Design review of the part built by this model. Coordinates are the model's own, in mm. A direction names the side the tool comes from. Coordinates: 2 decimals unless noted, no trailing zeros. Write each loop counter-clockwise with the first axis right and the second up, starting at its lowest first coordinate (ties: lowest second). Pieces come first, ordered by that corner, then holes. Notation, with made-up numbers: (-36, -20) - (-31, -20) arc R14 cw to (-31, -8) - close; hole circle Ø7 at (57.5, -1). An arc over 180 degrees is marked (long way). Use a Markdown table: item, result.
from build123d import *

# Parameters (mm, degrees)
SKETCH1_R               = 1.75
BOSS_EXTRUDE1_DEPTH     = 3
SKETCH2_R               = 2.1
BOSS_EXTRUDE2_DEPTH     = 10
SKETCH3_R               = 2.1
BOSS_EXTRUDE3_DEPTH     = 10
BOSS_EXTRUDE4_DEPTH     = 2
FILLET1_R               = 2
SKETCH6_R               = 2.1
CUT_EXTRUDE1_DEPTH      = 12
CUT_EXTRUDE1_DEPTH_BACK = 2.5
FILLET2_R               = 5


with BuildPart() as part:
    # Sketch1 → Boss-Extrude1 (new body)
    with BuildSketch(Plane.XY):
        with BuildLine():
            Line((-17, 23), (17, 23))
            Line((17, 23), (17, 13))
            Line((17, 13), (13.5, 13))
            ThreePointArc((13.5, 13), (9, 0), (13.5, -13))
            Line((13.5, -13), (17, -13))
            Line((17, -13), (17, -23))
            Line((17, -23), (-17, -23))
            Line((-17, -23), (-17, -13))
            Line((-17, -13), (-13.5, -13))
            ThreePointArc((-13.5, -13), (-9, 0), (-13.5, 13))
            Line((-13.5, 13), (-17, 13))
            Line((-17, 13), (-17, 23))
        make_face()
        Circle(SKETCH1_R, mode=Mode.SUBTRACT)
        with Locations((0, 17)):
            Circle(SKETCH1_R, mode=Mode.SUBTRACT)
        with Locations((-9.5, -17)):
            Circle(SKETCH1_R, mode=Mode.SUBTRACT)
        with Locations((9.5, -17)):
            Circle(SKETCH1_R, mode=Mode.SUBTRACT)
        with BuildLine():
            Line((-3.25, 13), (3.25, 13))
            ThreePointArc((3.25, 13), (5.194543648, 12.194543648), (6, 10.25))
            Line((6, 10.25), (6, 7.75))
            ThreePointArc((6, 7.75), (5.194543648, 5.805456352), (3.25, 5))
            Line((3.25, 5), (-3.25, 5))
            ThreePointArc((-3.25, 5), (-5.194543648, 5.805456352), (-6, 7.75))
            Line((-6, 7.75), (-6, 10.25))
            ThreePointArc((-6, 10.25), (-5.194543648, 12.194543648), (-3.25, 13))
        make_face(mode=Mode.SUBTRACT)
        with BuildLine():
            Line((-3.25, -5), (3.25, -5))
            ThreePointArc((3.25, -5), (5.194543648, -5.805456352), (6, -7.75))
            Line((6, -7.75), (6, -10.25))
            ThreePointArc((6, -10.25), (5.194543648, -12.194543648), (3.25, -13))
            Line((3.25, -13), (-3.25, -13))
            ThreePointArc((-3.25, -13), (-5.194543648, -12.194543648), (-6, -10.25))
            Line((-6, -10.25), (-6, -7.75))
            ThreePointArc((-6, -7.75), (-5.194543648, -5.805456352), (-3.25, -5))
        make_face(mode=Mode.SUBTRACT)
    extrude(amount=BOSS_EXTRUDE1_DEPTH)

    # Sketch2 → Boss-Extrude2 (add)
    with BuildSketch(Plane(origin=(0, 23, 0), x_dir=(1, 0, 0), z_dir=(0, 1, 0))):
        with BuildLine():
            Line((-20, -3), (-15.5, -3))
            Line((-15.5, -3), (-15.5, 1.5))
            ThreePointArc((-15.5, 1.5), (-23.181980515, 4.681980515), (-20, -3))
        make_face()
        with Locations((-20, 1.5)):
            Circle(SKETCH2_R, mode=Mode.SUBTRACT)
        with BuildLine():
            Line((20, -3), (15.5, -3))
            Line((15.5, -3), (15.5, 1.5))
            ThreePointArc((15.5, 1.5), (23.181980515, 4.681980515), (20, -3))
        make_face()
        with Locations((20, 1.5)):
            Circle(SKETCH2_R, mode=Mode.SUBTRACT)
    extrude(amount=-BOSS_EXTRUDE2_DEPTH)

    # Sketch3 → Boss-Extrude3 (add)
    with BuildSketch(Plane.XZ.offset(23)):
        with BuildLine():
            Line((-15.5, 3), (-20, 3))
            ThreePointArc((-20, 3), (-23.181980515, -4.681980515), (-15.5, -1.5))
            Line((-15.5, -1.5), (-15.5, 3))
        make_face()
        with Locations((-20, -1.5)):
            Circle(SKETCH3_R, mode=Mode.SUBTRACT)
        with BuildLine():
            Line((15.5, 3), (15.5, -1.5))
            ThreePointArc((15.5, -1.5), (23.181980515, -4.681980515), (20, 3))
            Line((20, 3), (15.5, 3))
        make_face()
        with Locations((20, -1.5)):
            Circle(SKETCH3_R, mode=Mode.SUBTRACT)
    extrude(amount=-BOSS_EXTRUDE3_DEPTH)

    # Sketch4 → Boss-Extrude4 (add)
    with BuildSketch(Plane(origin=(0, 23, 0), x_dir=(1, 0, 0), z_dir=(0, 1, 0))):
        with BuildLine():
            Line((-12.5, 0), (12.5, 0))
            Line((12.5, 0), (12.5, 8))
            ThreePointArc((12.5, 8), (11.621320344, 10.121320344), (9.5, 11))
            Line((9.5, 11), (-9.5, 11))
            ThreePointArc((-9.5, 11), (-11.621320344, 10.121320344), (-12.5, 8))
            Line((-12.5, 8), (-12.5, 0))
        make_face()
    extrude(amount=-BOSS_EXTRUDE4_DEPTH)

    # Fillet1
    fillet1_edges = [part.edges().sort_by_distance(p)[0] for p in [
        (-12.5, 22, 0),
        (0, 21, 0),
        (12.5, 22, 0),
    ]]
    fillet(fillet1_edges, radius=FILLET1_R)

    # Sketch6 → Cut-Extrude1 (cut, two sides)
    with BuildSketch(Plane(origin=(0, 0, 0), x_dir=(-1, 0, 0), z_dir=(0, 0, -1))) as cut_extrude1_sk:
        Circle(SKETCH6_R)
        with Locations((0, 17)):
            Circle(SKETCH6_R)
        with Locations((-9.5, -17)):
            Circle(SKETCH6_R)
        with Locations((9.5, -17)):
            Circle(SKETCH6_R)
    extrude(amount=CUT_EXTRUDE1_DEPTH, mode=Mode.SUBTRACT)
    extrude(cut_extrude1_sk.sketch, amount=-CUT_EXTRUDE1_DEPTH_BACK, mode=Mode.SUBTRACT)

    # Fillet2
    fillet2_edges = [part.edges().sort_by_distance(p)[0] for p in [
        (-13.5, -13, 1.5),
        (13.5, -13, 1.5),
        (-13.5, 13, 1.5),
        (13.5, 13, 1.5),
    ]]
    fillet(fillet2_edges, radius=FILLET2_R)


solid = part.part
(1) For pin 1 (2 mm diameter, centred on x = 3.5, y = 13.5, fed in from -Z); pin 2 (0.6 mm diameter, centred on y = 22.5, z = -5, fed in from -X); pin 3 (4 mm diameter, centred on x = 9.5, y = -17, fed in from -Z); pin 4 (2 mm diameter, centred on x = 0, y = 17, fed in from +Z), all flat-tipped, find the tip position at first contact; note any pin that passes through.
Determined:
| item | result |
|---|---|
| pin 1 | z = 0 |
| pin 2 | x = -23.16 |
| pin 3 | z = 2.5 |
| pin 4 | through |
(2) Draft analysis for pull direction X (two halves, no side actions). For faces 6 (the cylindrical face through (13.605, 12.31, 1.155)), 7 (the cylindrical face through (-13.605, -12.31, 1.155)), 8 (the cylindrical face through (-1.13, 18.77, 1.23)), state which applies: +X half, -X half, draft (parallel to the pull), parting line (faces both ways), or undercut.
Determined:
| item | result |
|---|---|
| face 6 | +X half |
| face 7 | -X half |
| face 8 | undercut |
(3) For L1, parallel to Y at x = 0, z = 2.8; L2, parallel to X at y = 0, z = 2.6; L3, parallel to Z at x = -20, y = -15.75, list the stretches that pass through material, from the lowest coordinate up. Write a range as from..to.
Determined:
| item | result |
|---|---|
| L1 | -23..-13, -5..-1.75, 1.75..5, 13..15.25, 18.75..23 |
| L2 | -9..-1.75, 1.75..9 |
| L3 | -6..-3.6, 0.6..3 |
(4) Take a section at D-D on z = -4.75. Write out the cut boundary in (x, y).
Determined:
| item | result |
|---|---|
| outline | (-23.11, -23) - (-16.89, -23) - (-16.89, -13) - (-23.11, -13) - close; (-23.11, 13) - (-16.89, 13) - (-16.89, 23) - (-23.11, 23) - close; (-12.5, 21) - (12.5, 21) - (12.5, 23) - (-12.5, 23) - close; (16.89, -23) - (23.11, -23) - (23.11, -13) - (16.89, -13) - close; (16.89, 13) - (23.11, 13) - (23.11, 23) - (16.89, 23) - close |
(5) Take a section at B-B on x = 0. State how many separate pieces and enclosed holes the cut face has, and give its area (3 significant figures).
Determined:
| item | result |
|---|---|
| separate pieces | 5 |
| enclosed holes | 0 |
| area | 88.4 mm2 |
(6) Take a section at C-C on y = 16. Write out the cut boundary in (x, z), and give its area (3 significant figures).
Determined:
| item | result |
|---|---|
| outline | (-20, 3) arc R4.5 ccw (long way) to (-15.5, -1.5) - (-15.5, 0) - (-1.85, 0) - (-1.85, 2.5) - (-1.44, 2.5) - (-1.44, 3) - close; (1.44, 2.5) - (1.85, 2.5) - (1.85, 0) - (15.5, 0) - (15.5, -1.5) arc R4.5 ccw (long way) to (20, 3) - (1.44, 3) - close; hole circle Ø4.2 at (-20, -1.5); hole circle Ø4.2 at (20, -1.5) |
| area | 191 mm2 |
(7) Machinability: for faces 1 (the flat face through (0, 22, -11)), 2 (the cylindrical face through (-13.67, 12.35, 1.16)), 3 (the cylindrical face through (13.67, -12.35, 1.16)), 4 (the flat face through (6, 9, 1)), 5 (the cylindrical face through (-13.37, 21.42, -0.35)), which of the approach directions +Z, -Z, +X, -X, +Y, -Y give a long, thin tool a straight path to every point of the face, cutting with its end or side? Answer none if there is none.
Determined:
| item | result |
|---|---|
| face 1 | -Z, +X, -X, +Y, -Y |
| face 2 | +Z, -Z, -X |
| face 3 | +Z, -Z, +X |
| face 4 | +Z, -Z |
| face 5 | -Z, +Y, -Y |
(8) Take a section at A-A on y = -17. Write out the cut boundary in (x, z), and give its area (3 significant figures).
Determined:
| item | result |
|---|---|
| outline | (-20, 3) arc R4.5 ccw (long way) to (-15.5, -1.5) - (-15.5, 0) - (-11.6, 0) - (-11.6, 2.5) - (-11.25, 2.5) - (-11.25, 3) - close; (-7.75, 2.5) - (-7.4, 2.5) - (-7.4, 0) - (7.4, 0) - (7.4, 2.5) - (7.75, 2.5) - (7.75, 3) - (-7.75, 3) - close; (11.25, 2.5) - (11.6, 2.5) - (11.6, 0) - (15.5, 0) - (15.5, -1.5) arc R4.5 ccw (long way) to (20, 3) - (11.25, 3) - close; hole circle Ø4.2 at (-20, -1.5); hole circle Ø4.2 at (20, -1.5) |
| area | 177 mm2 |
